Autodesk Inventor part; units mm, degrees
ref_plane "YZ Plane" through (0, 0, 0) normal (1, 0, 0) x (0, 1, 0)
ref_plane "XZ Plane" through (0, 0, 0) normal (0, 1, 0) x (-1, 0, 0)
ref_plane "XY Plane" through (0, 0, 0) normal (0, 0, 1) x (1, 0, 0)
sketch "Sketch1" plane through (0, 0, 0) normal (0, 0, 1) x (1, 0, 0)
  circle A0 centre (0, 0) radius 3.5
  circle A1 centre (0, 0) radius 4.5
  dimension "d0" = 7
  dimension "d1" = 9
extrude "Extrusion1" add sketch "Sketch1" along normal blind 6
sketch "Sketch2" plane through (0, 0, 0) normal (0, 0, -1) x (-1, 0, 0)
  circle A0 centre (0, 0) radius 1.5
  circle A1 centre (0, 0) radius 5.5
  dimension "d4" = 3
  dimension "d5" = 11
extrude "Extrusion2" add sketch "Sketch2" along normal blind 2
properties part number "cork"
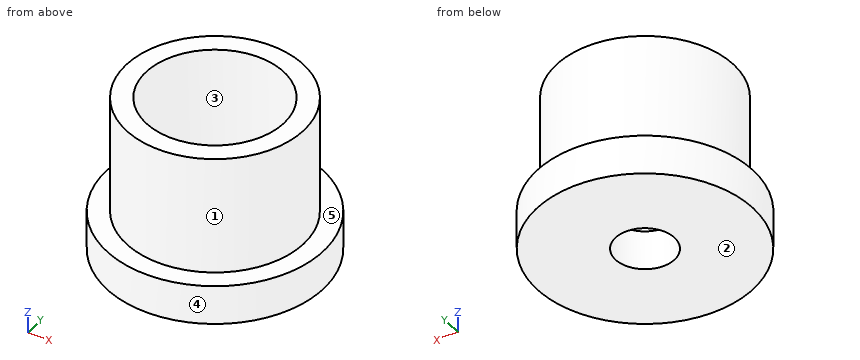
Can you work these out from the model? Positions are in its coordinate system, mm. Face numbers are marked on the shaded views. A direction names the side the tool comes from. Coordinates: 2 decimals unless noted, no trailing zeros. Loops run counter-clockwise (first coordinate to the right, second up) from the corner with the lowest first, then second, coordinate; pieces in that order, holes last. Notation, with made-up numbers: (68.5, -34.5) -> (112.5, -34.5) arc R25 cw to (112.5, -15.5) -> close; hole circle Ø5 at (-34, 31). An arc over 180 degrees is marked (long way). Answer as a JSON object with one key per item and string values.
1) Imagine slicing it at A-A (y = 0). Please give me the cut outline in (x, z), then the cut area to 3 significant figures.
Results:
{"outline": "(-5.5, -2) -> (-1.5, -2) -> (-1.5, 0) -> (-3.5, 0) -> (-3.5, 6) -> (-4.5, 6) -> (-4.5, 0) -> (-5.5, 0) -> close; (1.5, -2) -> (5.5, -2) -> (5.5, 0) -> (4.5, 0) -> (4.5, 6) -> (3.5, 6) -> (3.5, 0) -> (1.5, 0) -> close", "area": "28.0 mm^2"}
2) If I drill on line 1 (Y direction, x = 0, z = 1.25); line 2 (X direction, y = 3, z = 1.75); line 3 (Z direction, x = 1.25, y = 2), over which ranges is the centre line in solid material (lowest first)?
Results:
{"line 1": "y = -4.5 to -3.5, 3.5 to 4.5", "line 2": "x = -3.35 to -1.8, 1.8 to 3.35", "line 3": "z = -2 to 0"}
3) Imagine slicing it at C-C (x = 3.75). Please give me the cut outline in (y, z).
Results:
{"outline": "(-4.02, -2) -> (4.02, -2) -> (4.02, 0) -> (2.49, 0) -> (2.49, 6) -> (-2.49, 6) -> (-2.49, 0) -> (-4.02, 0) -> close"}
4) For the marked faces 4 and 5, which set-ups out of +Z, -Z, +X, -X, +Y, -Y let a thin tool reach every point of the face, with its end or its side?
Results:
{"face 4": "+Z, -Z", "face 5": "+Z"}
5) For P1, Ø1, axis at y = 4, z = 1.5, coming from the -X side; P2, Ø1, axis at y = -4, z = 5, coming from the +X side; P3, Ø2, axis at x = -0.5, z = 5, coming from the -Y side, each with a flat end and sliding along its axis, tell me the tip position at first contact or that it passes through.
Results:
{"P1": "stops at x = -2.83", "P2": "stops at x = 2.83", "P3": "stops at y = -4.5"}
6) Thinking about a two-plate mould opening in X: for the marked faces 1, 2 and 3, which applies, pulls with the +X half, pulls with the -X half, needs draft (parallel to the pull), parting line crosses it, or undercut?
Results:
{"face 1": "parting line crosses it", "face 2": "needs draft", "face 3": "undercut"}
7) Imagine slicing it at D-D (z = 3). Please give me the cut outline in (x, y).
Results:
{"outline": "circle Ø9 at (0, 0); hole circle Ø7 at (0, 0)"}
